Autodesk Inventor part; units mm, degrees
ref_plane "YZ Plane" through (0, 0, 0) normal (1, 0, 0) x (0, 1, 0)
ref_plane "XZ Plane" through (0, 0, 0) normal (0, 1, 0) x (-1, 0, 0)
ref_plane "XY Plane" through (0, 0, 0) normal (0, 0, 1) x (1, 0, 0)
sketch "Sketch1" plane through (0, 0, 0) normal (0, 0, 1) x (1, 0, 0)
  circle A0 centre (0, 0) radius 2.7432
  dimension "d0" = 5.4864
extrude "Extrusion1" add sketch "Sketch1" against normal blind 9.525
sketch "Sketch2" plane through (0, 0, -9.525) normal (0, 0, -1) x (-1, 0, 0)
  circle A0 centre (0, 0) radius 1.7907
  dimension "d3" = 3.5814
extrude "Extrusion2" add sketch "Sketch2" along normal blind 9.525
thread "Thread1"
thread "Thread2"
sketch "Sketch3" plane through (0, 0, 0) normal (0, 0, 1) x (1, 0, 0)
  line L0 (0, 0) -> (0, 3.3215) construction
  line L1 (-0.3969, 2.772) -> (0.3969, 2.772)
  line L2 (0.3969, 2.772) -> (0.3969, 0)
  line L3 (0.3969, 0) -> (-0.3969, 0)
  line L4 (-0.3969, 0) -> (-0.3969, 2.772)
  dimension "d10" = 0.3969
  dimension "d11" = 0.7937
extrude "Extrusion3" cut sketch "Sketch3" against normal blind 1.1906
properties part number "VS-010 (SET SCREW)" material "Steel, Carbon"
The model under review builds one solid part; all positions refer to its coordinate system, in mm. A direction names the side the tool comes from. Round coordinates to 2 decimals unless told otherwise and drop trailing zeros. Write each loop counter-clockwise with the first axis right and the second up, starting at its lowest first coordinate (ties: lowest second). Pieces come first, ordered by that corner, then holes. Notation, with made-up numbers: M 4,48.25 L 31,48.25 A31 ccw 31,87.25 Z; hole C 46.5,-26.5 d2. An arc over 180 degrees is marked long. Answer as CSV lines item,"result". Start each with the question number.
Q1. Tool access review of faces 1 (the face through (0, 0, -19.05)), 2 (the face through (0.388, 1.748, -14.221)): name each direction out of +Z, -Z, +X, -X, +Y, -Y from which nothing blocks a thin tool from reaching the whole face with its end or side.
Q2. The part is to be moulded in two halves that separate along X. For faces 3 (the face through (-0.397, 1, -1)), 4 (the face through (0.397, 1, -1)), 5 (the face through (0, -1, 0)), 6 (the face through (-0.59, -2.68, -4.7)), say which applies: +X half, -X half, draft (parallel to the pull), parting line (faces both ways), or undercut.
Q3. Clearance check with flat-ended pins moving along their axes: P1, Ø2, axis at x = 2, y = -1.5, coming from the +Z side; P2, Ø1.5, axis at y = 2, z = -4, coming from the -X side; P3, Ø1, axis at y = 2, z = -0.5, coming from the +X side; P4, Ø2, axis at x = -2, z = -13, coming from the +Y side. State where each tip first meets the part, or that it passes through.
Q4. Consider section C-C, the plane z = -11. Give the boundary of the cut face in (x, y), then the cut area to 3 significant figures.
Q5. Wall thickness on line 1 along Z through (x, y) = (-0.1, 2.25) (3 decimals); line 2 along Z through (x, y) = (-0.3, 0.25); line 3 along X through (y, z) = (1.3, -10.25): over which ranges is each line inside the solid? List them lowest first.
Q6. Consider section A-A, the plane x = 0. Give the boundary of the cut face in (y, z) (3 decimals).
Q7. Consider section B-B, the plane y = 0.6. Give the boundary of the cut face in (x, z) (3 decimals), then the cut area to 3 significant figures.
Q8. Consider section D-D, the plane z = -6.5. Give the boundary of the cut face in (x, y), then the cut area to 3 significant figures.
Result set:
1,face 1,"-Z, +X, -X, +Y, -Y"
1,face 2,"-Z"
2,face 3,"undercut"
2,face 4,"undercut"
2,face 5,"draft"
2,face 6,"parting line"
3,P1,"stops at z = 0"
3,P2,"stops at x = -2.44"
3,P3,"stops at x = 2.3"
3,P4,"stops at y = 1.49"
4,outline,"C 0,0 d3.58"
4,area,"10.1 mm²"
5,line 1,"z = -9.525 to -1.191"
5,line 2,"z = -19.05 to -1.19"
5,line 3,"x = -1.23 to 1.23"
6,outline,"M -2.743,-9.525 L -1.791,-9.525 L -1.791,-19.05 L 1.791,-19.05 L 1.791,-9.525 L 2.743,-9.525 L 2.743,-1.191 L 0,-1.191 L 0,0 L -2.743,0 Z"
7,outline,"M -2.677,-9.525 L -1.687,-9.525 L -1.687,-19.05 L 1.687,-19.05 L 1.687,-9.525 L 2.677,-9.525 L 2.677,0 L 0.397,0 L 0.397,-1.191 L -0.397,-1.191 L -0.397,0 L -2.677,0 Z"
7,area,"82.2 mm²"
8,outline,"C 0,0 d5.49"
8,area,"23.6 mm²"
